from build123d import *

# Parameters (mm, degrees)
F0_W     = 43.2927459478
F0_H     = 35.019159317
F1_DEPTH = 50.8
F2_R     = 10
F3_R     = 10
F4_SIZE  = 5.08
F5_SIZE  = 5.08
F6_SIZE  = 5.08


with BuildPart() as f1:
    # F0 (on Top) → F1 (new body)
    with BuildSketch(Plane.XY):
        with Locations((-21.6463729739, 17.5095796585)):
            Rectangle(F0_W, F0_H)
    extrude(amount=F1_DEPTH)

    # F2
    f2_edges = [f1.edges().sort_by_distance(p)[0] for p in [
        (-43.292746, 17.50958, 50.8),
    ]]
    fillet(f2_edges, radius=F2_R)

    # F3
    f3_edges = [f1.edges().sort_by_distance(p)[0] for p in [
        (-43.292746, 17.50958, 0),
    ]]
    fillet(f3_edges, radius=F3_R)

    # F4
    f4_edges = [f1.edges().sort_by_distance(p)[0] for p in [
        (0, 17.50958, 0),
    ]]
    chamfer(f4_edges, length=F4_SIZE)

    # F5
    f5_edges = [f1.edges().sort_by_distance(p)[0] for p in [
        (0, 17.50958, 50.8),
    ]]
    chamfer(f5_edges, length=F5_SIZE)

    # F6
    f6_edges = [f1.edges().sort_by_distance(p)[0] for p in [
        (-2.54, 35.019159, 2.54),
        (-19.186373, 35.019159, 50.8),
        (0, 35.019159, 25.4),
        (-40.363814, 35.019159, 47.871068),
        (-19.186373, 35.019159, 0),
        (-2.54, 35.019159, 48.26),
        (-40.363814, 35.019159, 2.928932),
        (-43.292746, 35.019159, 25.4),
    ]]
    chamfer(f6_edges, length=F6_SIZE)


solid = f1.part
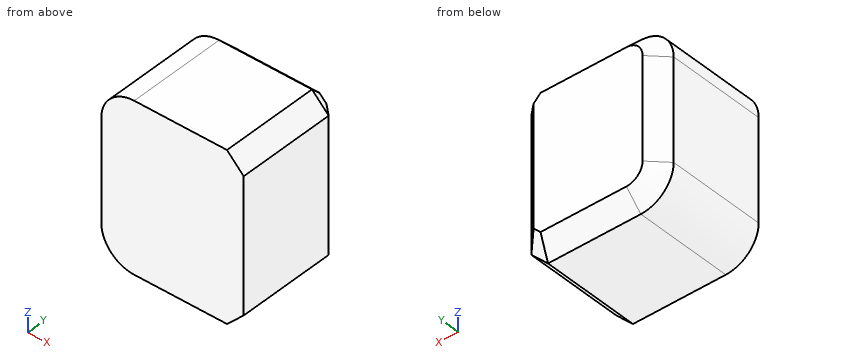
Verification items for the finished model (mm, model axes). Round coordinates to 2 decimals unless told otherwise and drop trailing zeros. Loops run counter-clockwise (first coordinate to the right, second up) from the corner with the lowest first, then second, coordinate; pieces in that order, holes last. Notation, with made-up numbers: (54, 9.25) - (70, 9.25) arc R23 cw to (70, 21.25) - close; hole circle Ø7 at (-35.75, -5). An arc over 180 degrees is marked (long way). Use a Markdown table: item, result. Add a question column.
1. Section check D-D, the plane y = 31. Record the boundary of the cut face in (x, z), plus the area to 3 significant figures.
2. Section check C-C, the plane x = -3.5. Record the boundary of the cut face in (y, z).
3. Gauge pin test, flat end, axial feed: pin 1 (5 mm diameter, centred on x = -36, y = 25.5, fed in from +Z). Record the tip position at first contact, or that the pin passes through.
4. Section check B-B, the plane z = 37.5. Record the boundary of the cut face in (x, y).
5. Thickness scan on probe 1 along Z at (x, y) = (-27.5, 30); probe 2 along X at (y, z) = (24.5, 47); probe 3 along Z at (x, y) = (-25, 31). Record the ranges inside material, lowest first. Write a range as [from, to].
6. Section check A-A, the plane y = 26.5. Record the boundary of the cut face in (x, z).
Checks:
| question | item | result |
|---|---|---|
| 1 | outline | (-42.23, 10) arc R8.94 ccw to (-33.29, 1.06) - (-5.52, 1.06) - (-1.06, 5.52) - (-1.06, 45.28) - (-5.52, 49.74) - (-33.29, 49.74) arc R8.94 ccw to (-42.23, 40.8) - close |
| 1 | area | 1,950 mm^2 |
| 2 | outline | (0, 1.58) - (29.94, 1.58) - (33.44, 6.53) - (33.44, 44.27) - (29.94, 49.22) - (0, 49.22) - close |
| 3 | pin 1 | stops at z = 50.8 |
| 4 | outline | (-43.29, 0) - (0, 0) - (0, 29.94) - (-5.08, 35.02) - (-38.21, 35.02) - (-43.29, 29.94) - close |
| 5 | probe 1 | z = [0.06, 50.74] |
| 5 | probe 2 | x = [-41.14, -1.28] |
| 5 | probe 3 | z = [1.06, 49.74] |
| 6 | outline | (-43.29, 10) arc R10 ccw to (-33.29, 0) - (-5.08, 0) - (0, 5.08) - (0, 45.72) - (-5.08, 50.8) - (-33.29, 50.8) arc R10 ccw to (-43.29, 40.8) - close |
